Autodesk Inventor part; units mm, degrees
ref_plane "YZ Plane" through (0, 0, 0) normal (1, 0, 0) x (0, 1, 0)
ref_plane "XZ Plane" through (0, 0, 0) normal (0, 1, 0) x (-1, 0, 0)
ref_plane "XY Plane" through (0, 0, 0) normal (0, 0, 1) x (1, 0, 0)
sketch "Sketch1" plane through (0, 0, 0) normal (0, 1, 0) x (-1, 0, 0)
  arc A0 (19.05, -12.7) -> (19.05, 12.7) centre (19.05, 0) ccw
  arc A1 (-21.2006, 12.7) -> (-21.2006, -12.7) centre (-31.75, 0) ccw
  circle A2 centre (-31.75, 0) radius 10.9982
  circle A3 centre (19.05, 0) radius 7.9375
  line L0 (19.05, -12.7) -> (-24.3756, -12.7)
  line L1 (19.05, 12.7) -> (-24.3756, 12.7)
  line L2 (-31.75, 0) -> (19.05, 0)
  point P0 (0, 0)
  point P1 (-21.2006, 12.7)
  dimension "d4" = 15.875
  dimension "d9" = 50.8
extrude "Extrusion1" add sketch "Sketch1" along normal blind 7.1374
properties part number "Connecting Rod"
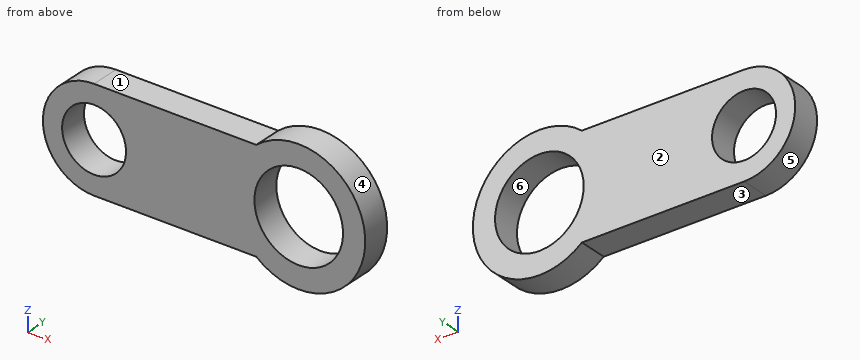
Verification items for the finished model (mm, model axes). Face numbers are marked on the shaded views. A direction names the side the tool comes from. Coordinates: 2 decimals unless noted, no trailing zeros. Loops run counter-clockwise (first coordinate to the right, second up) from the corner with the lowest first, then second, coordinate; pieces in that order, holes last. Notation, with made-up numbers: (48.5, 37.5) - (80.5, 37.5) arc R20 ccw to (80.5, 70.5) - close; hole circle Ø8 at (21, 7). An arc over 180 degrees is marked (long way). Return JSON: item names as keys, results as strings.
1. Thickness scan on L1, parallel to X at y = 3.25, z = -6.5; L2, parallel to Z at x = -19.05, y = 4; L3, parallel to Z at x = 31.75, y = 2.25. Record the ranges inside material, lowest first.
Established:
{"L1": "x = -29.96 to -23.61, -14.49 to 22.88, 40.62 to 46.93", "L2": "z = -12.7 to -7.94, 7.94 to 12.7", "L3": "z = -16.51 to -11, 11 to 16.51"}
2. Section check B-B, the plane x = 31.75. Record the boundary of the cut face in (y, z), then the cut area to 3 significant figures.
Established:
{"outline": "(0, -16.51) - (7.14, -16.51) - (7.14, -11) - (0, -11) - close; (0, 11) - (7.14, 11) - (7.14, 16.51) - (0, 16.51) - close", "area": "78.7 mm2"}
3. Section check C-C, the plane y = 1. Count the separate pieces of the cut face and the enclosed holes in it, then the cut area to 3 significant figures.
Established:
{"separate pieces": "1", "enclosed holes": "2", "area": "1,450 mm2"}
4. Mould release check, pull along X, two halves, no side actions. Record for the marked faces 3, 4, 5 and 6: +X half, -X half, draft (parallel to the pull), parting line (faces both ways), or undercut.
Established:
{"face 3": "draft", "face 4": "parting line", "face 5": "-X half", "face 6": "undercut"}
5. Section check D-D, the plane z = 10. Record the boundary of the cut face in (x, y), then the cut area to 3 significant figures.
Established:
{"outline": "(-26.88, 0) - (27.17, 0) - (27.17, 7.14) - (-26.88, 7.14) - close; (36.33, 0) - (44.89, 0) - (44.89, 7.14) - (36.33, 7.14) - close", "area": "447 mm2"}
6. Section check A-A, the plane z = 0. Record the boundary of the cut face in (x, y).
Established:
{"outline": "(-31.75, 0) - (-26.99, 0) - (-26.99, 7.14) - (-31.75, 7.14) - close; (-11.11, 0) - (20.75, 0) - (20.75, 7.14) - (-11.11, 7.14) - close; (42.75, 0) - (48.26, 0) - (48.26, 7.14) - (42.75, 7.14) - close"}
7. Tool access check on the marked faces 1 and 2. Record the directions out of +Z, -Z, +X, -X, +Y, -Y that give a thin tool (end or side, any length) a straight path to the whole face; none if there is none.
Established:
{"face 1": "+Z, -X, +Y, -Y", "face 2": "+Z, -Z, +X, -X, +Y"}
8. Go/stop test with flat-tipped pins: pin 1 (3 mm diameter, centred on x = 25, z = -5.5, fed in from -Y); pin 2 (2 mm diameter, centred on y = 3.5, z = -4, fed in from +X); pin 3 (1 mm diameter, centred on x = 5.5, y = 1.5, fed in from -Z); pin 4 (1.5 mm diameter, centred on y = 1.5, z = -2, fed in from -X). Record where each tip stops, or that it passes through.
Established:
{"pin 1": "passes through", "pin 2": "stops at x = 47.99", "pin 3": "stops at z = -12.7", "pin 4": "stops at x = -31.69"}
